Read the model definition and answer for the solid it produces. Units are mm, in the model's axes. A direction names the side the tool comes from. Give positions to 0.01 mm unless a question says otherwise; leave off trailing zeros. Loops run counter-clockwise (first coordinate to the right, second up) from the corner with the lowest first, then second, coordinate; pieces in that order, holes last. Notation, with made-up numbers: (10.25, 68) -> (31.25, 68) arc R23 ccw to (31.25, 94) -> close; hole circle Ø9 at (50.5, 4). An arc over 180 degrees is marked (long way). Write each question's results on one line, items separated by ' | '. Start each with the question number.
Item 1: Find the intervals of material crossed by line 1 (Z direction, x = 41, y = -3); line 2 (X direction, y = -3.5, z = 22); line 3 (Y direction, x = -5, z = 2.5), in increasing order.
Item 2: Each of these flat-tipped pins is pushed along its axis until it touches: P1, Ø1.5, axis at y = 52.5, z = 5.5, coming from the -X side; P2, Ø10, axis at x = 8, z = 27, coming from the +Y side; P3, Ø10, axis at y = -60.5, z = 9.5, coming from the -X side. Where does it stop, or does it pass through?
Item 3: Which of the six approach directions +Z, -Z, +X, -X, +Y, -Y give full straight-line access (tool end or side, diameter ignored) to faces 1 (the flat face through (69.14, -29.07, 4.93)), 2 (the cylindrical face through (-1.08, -4.88, 19.86))?
Item 4: Section A-A on x = 0 is taken. Write down the section's boundary in (y, z), and give its area (3 significant figures).
Item 5: Section B-B on z = 3.5 is taken. Write down the section's boundary in (x, y), and give its area (3 significant figures).
Item 6: Section D-D on z = 24 is taken. Write down the section's boundary in (x, y), and give its area (3 significant figures).
```python
from build123d import *

# Parameters (mm, degrees)
F1_DEPTH = 10
F2_R     = 5
F3_DEPTH = 20
F4_R     = 7


with BuildPart() as f1:
    # F0 (on Top) → F1 (new body)
    with BuildSketch(Plane.XY):
        Polygon((81.179415, 0), (57.402515, 57.402515), (0, 81.179415), (-57.402515, 57.402515), (-81.179415, 0), (-57.402515, -57.402515), (0, -81.179415), (57.402515, -57.402515), align=None)
    extrude(amount=F1_DEPTH)

    # F2 (on face) → F3 (join)
    with BuildSketch(Plane.XY.offset(10)):
        Circle(F2_R)
    extrude(amount=F3_DEPTH)

    # F4
    f4_edges = [f1.edges().sort_by_distance(p)[0] for p in [
        (-57.402515, 57.402515, 5),
        (-81.179415, 0, 5),
        (0, 81.179415, 5),
        (-57.402515, -57.402515, 5),
        (0, -81.179415, 5),
        (57.402515, -57.402515, 5),
        (81.179415, 0, 5),
        (57.402515, 57.402515, 5),
    ]]
    fillet(f4_edges, radius=F4_R)


solid = f1.part
```
Findings:
1) line 1: 0 to 10 | line 2: -3.57 to 3.57 | line 3: -79.11 to 79.11
2) P1: x = -59.74 | P2: y = 4 | P3: x = -58.13
3) face 1: +Z, -Z, +X, -Y | face 2: +Z
4) outline: (-80.6, 0) -> (80.6, 0) -> (80.6, 10) -> (5, 10) -> (5, 30) -> (-5, 30) -> (-5, 10) -> (-80.6, 10) -> close | area: 1,810 mm2
5) outline: (-80.07, -2.68) -> (-58.51, -54.72) arc R7 ccw to (-54.72, -58.51) -> (-2.68, -80.07) arc R7 ccw to (2.68, -80.07) -> (54.72, -58.51) arc R7 ccw to (58.51, -54.72) -> (80.07, -2.68) arc R7 ccw to (80.07, 2.68) -> (58.51, 54.72) arc R7 ccw to (54.72, 58.51) -> (2.68, 80.07) arc R7 ccw to (-2.68, 80.07) -> (-54.72, 58.51) arc R7 ccw to (-58.51, 54.72) -> (-80.07, 2.68) arc R7 ccw to start | area: 18,600 mm2
6) outline: circle Ø10 at (0, 0) | area: 78.5 mm2
